Can you work these out from the drawing? Everything is in mm from the part's minimum corner. A direction names the side the tool comes from. Give positions to 0.01 mm unless a question says otherwise; leave off trailing zeros. Write each loop counter-clockwise with the first axis right and the second up, starting at its lowest first coordinate (ties: lowest second). Pieces come first, ordered by that corner, then holes. Notation, with made-up numbers: (51, 74) -> (60, 74) arc R29 cw to (60, 95) -> close; hole circle Ø5 at (85.5, -21). An arc over 180 degrees is marked (long way). Use one line per item in the form item = value.
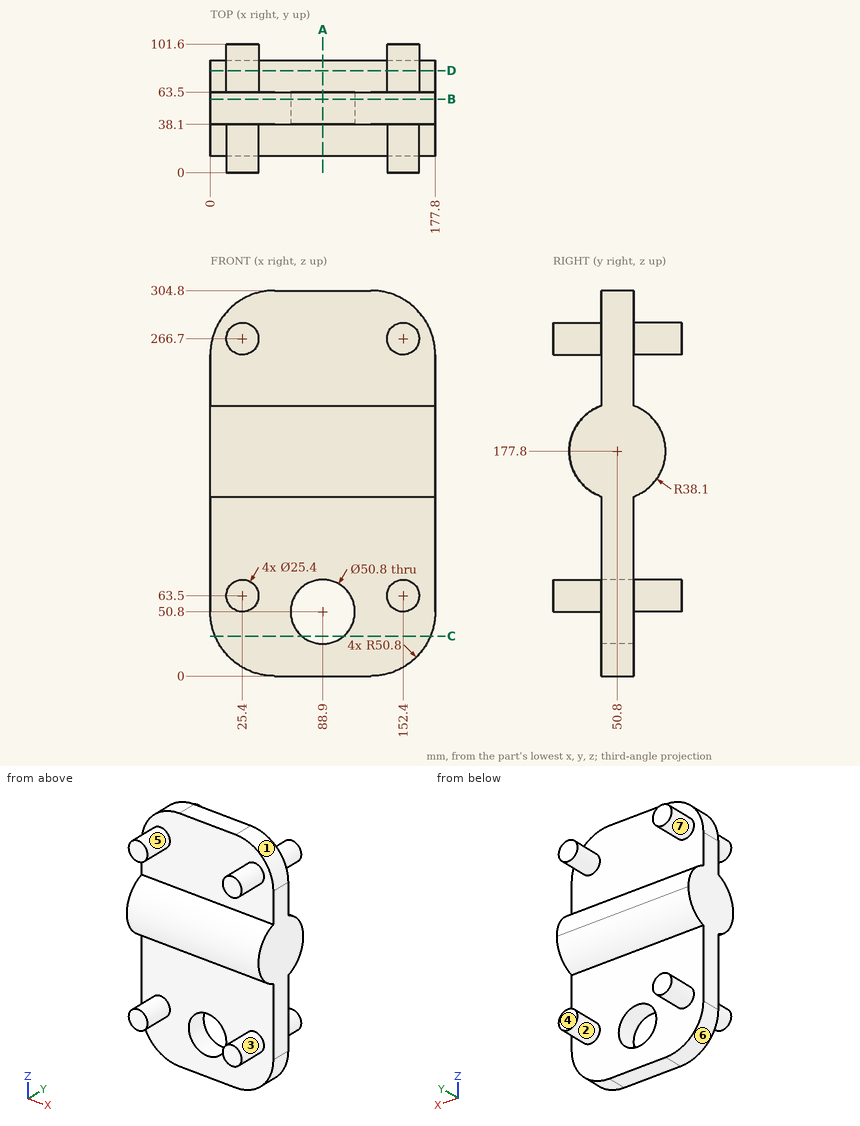
Q1. If we mould it in two halves opening along X, with no side actions, what happens to the marked faces 4, 5, 6 and 7? For each: +X half, -X half, draft (parallel to the pull), parting line (faces both ways), or undercut.
Result set:
face_4 = draft
face_5 = undercut
face_6 = -X half
face_7 = undercut
Q2. Which directions (+Z, -Z, +X, -X, +Y, -Y) give clear straight access to the entire face, cutting with the end or side of a thin tool? Please do the marked faces 1, 2 and 3.
Result set:
face_1 = +Z, +X, +Y, -Y
face_2 = +Y
face_3 = -Y
Q3. Will these pins go through, and if not, where does the flat tip stop? pin 1 Ø10 at (x, y) = (134, 72.5) entering from +Z (3 decimals); pin 2 Ø12 at (y, z) = (73.5, 61) entering from +X; pin 3 Ø1.5 at (x, z) = (136.5, 242.5) entering from +Y.
Result set:
pin_1 = 212.045
pin_2 = 165.1
pin_3 = 63.5
Q4. I want a section at A-A, the plane x = 88.9. Write out the boundary of the cut face in (y, z).
Result set:
outline = (38.1, 0) -> (63.5, 0) -> (63.5, 25.4) -> (38.1, 25.4) -> close; (38.1, 76.2) -> (63.5, 76.2) -> (63.5, 141.88) arc R38.1 ccw to (63.5, 213.72) -> (63.5, 304.8) -> (38.1, 304.8) -> (38.1, 213.72) arc R38.1 ccw to (38.1, 141.88) -> close
Q5. I want a section at D-D, the plane y = 80.5. Write out the boundary of the cut face in (x, z), and give its area (3 significant figures).
Result set:
outline = (0, 153.94) -> (177.8, 153.94) -> (177.8, 201.66) -> (0, 201.66) -> close; circle Ø25.4 at (25.4, 63.5); circle Ø25.4 at (25.4, 266.7); circle Ø25.4 at (152.4, 63.5); circle Ø25.4 at (152.4, 266.7)
area = 10,500 mm2
Q6. If I drill on line 1 along Z through (x, y) = (88.9, 58.5); line 2 along X through (y, z) = (51, 50); line 3 along Y through (x, z) = (156.5, 36), over which ranges is the centre line in solid material (lowest first)? Write a range as from..to.
Result set:
line_1 = 0..25.4, 76.2..304.8
line_2 = 0.01..63.51, 114.29..177.79
line_3 = 38.1..63.5
Q7. I want a section at B-B, the plane y = 58. Write out the boundary of the cut face in (x, z).
Result set:
outline = (0, 50.8) arc R50.8 ccw to (50.8, 0) -> (127, 0) arc R50.8 ccw to (177.8, 50.8) -> (177.8, 254) arc R50.8 ccw to (127, 304.8) -> (50.8, 304.8) arc R50.8 ccw to (0, 254) -> close; hole circle Ø50.8 at (88.9, 50.8)
Q8. I want a section at C-C, the plane z = 31.5. Write out the boundary of the cut face in (x, y), and give its area (3 significant figures).
Result set:
outline = (3.81, 38.1) -> (72.39, 38.1) -> (72.39, 63.5) -> (3.81, 63.5) -> close; (105.41, 38.1) -> (173.99, 38.1) -> (173.99, 63.5) -> (105.41, 63.5) -> close
area = 3,480 mm2
